For this review, take the finished solid that the model builds, in its own axes (mm). Face numbers are marked on the shaded views. A direction names the side the tool comes from. Round coordinates to 2 decimals unless told otherwise and drop trailing zeros. Order: outer loops, then holes, each group sorted by start corner. A loop starts at its lowest first (then second) coordinate and runs counter-clockwise, first axis right, second up.
from build123d import *

# Parameters (mm, degrees)
SKETCH1_W           = 26
SKETCH1_H           = 45
BOSS_EXTRUDE1_DEPTH = 11
SKETCH2_R           = 8.45
CUT_EXTRUDE1_DEPTH  = 28
CUT_EXTRUDE2_DEPTH  = 26.5
SKETCH5_W           = 6
SKETCH5_H           = 3
CUT_EXTRUDE3_DEPTH  = 53.509522946
BOSS_EXTRUDE4_START = 19
BOSS_EXTRUDE4_DEPTH = 19
SKETCH8_W           = 16
SKETCH8_H           = 16
CUT_EXTRUDE7_DEPTH  = 1.95
SKETCH9_W           = 6
SKETCH9_H           = 3
CUT_EXTRUDE8_DEPTH  = 53.502404707
SKETCH10_R          = 2
CUT_EXTRUDE9_DEPTH  = 4
SKETCH11_R          = 1.3
BOSS_EXTRUDE5_DEPTH = 26
SKETCH13_W          = 22
SKETCH13_H          = 12.79225404
CUT_EXTRUDE11_DEPTH = 54.122499941


with BuildPart() as part:
    # Sketch1 → Boss-Extrude1 (new body)
    with BuildSketch(Plane.XY):
        with Locations((13, -22.5)):
            Rectangle(SKETCH1_W, SKETCH1_H)
    extrude(amount=BOSS_EXTRUDE1_DEPTH)

    # Sketch2 → Cut-Extrude1 (cut)
    with BuildSketch(Plane.XZ.offset(45)):
        with Locations((13, -5.95)):
            Circle(SKETCH2_R)
    extrude(amount=-CUT_EXTRUDE1_DEPTH, mode=Mode.SUBTRACT)

    # Sketch4 → Cut-Extrude2 (cut)
    with BuildSketch(Plane(origin=(0, -43.5, 0), x_dir=(-1, 0, 0), z_dir=(0, -1, 0))):
        with BuildLine():
            Line((-1, -11), (-1, -1))
            Line((-1, -1), (-6.596875763, -1))
            ThreePointArc((-6.596875763, -1), (-13, -3.5), (-19.403124237, -1))
            Line((-19.403124237, -1), (-25, -1))
            Line((-25, -1), (-25, -11))
            Line((-25, -11), (-1, -11))
        make_face()
    extrude(amount=-CUT_EXTRUDE2_DEPTH, mode=Mode.SUBTRACT)

    # Sketch5 → Cut-Extrude3 (cut, through all)
    with BuildSketch(Plane.XY.offset(3.5)):
        with Locations((13, -26.5)):
            Rectangle(SKETCH5_W, SKETCH5_H)
    extrude(amount=-CUT_EXTRUDE3_DEPTH, mode=Mode.SUBTRACT)

    # Sketch6 → Boss-Extrude4 (add)
    with BuildSketch(Plane.XZ.offset(17).offset(BOSS_EXTRUDE4_START)):
        with BuildLine():
            Line((6.596875763, 1), (3.5, 1))
            Line((3.5, 1), (3.5, 5.5))
            Line((3.5, 5.5), (22.5, 5.5))
            Line((22.5, 5.5), (22.5, 1))
            Line((22.5, 1), (19.403124237, 1))
            ThreePointArc((19.403124237, 1), (13, 3.5), (6.596875763, 1))
        make_face()
    extrude(amount=-BOSS_EXTRUDE4_DEPTH)

    # Sketch8 → Cut-Extrude7 (cut)
    with BuildSketch(Plane.XY.offset(5.5)):
        with Locations((13, -26.5)):
            Rectangle(SKETCH8_W, SKETCH8_H)
    extrude(amount=-CUT_EXTRUDE7_DEPTH, mode=Mode.SUBTRACT)

    # Sketch9 → Cut-Extrude8 (cut, through all)
    with BuildSketch(Plane.XY.offset(3.55)):
        with Locations((13, -26.5)):
            Rectangle(SKETCH9_W, SKETCH9_H)
    extrude(amount=-CUT_EXTRUDE8_DEPTH, mode=Mode.SUBTRACT)

    # Sketch10 → Cut-Extrude9 (cut)
    with BuildSketch(Plane(origin=(26, 0, 0), x_dir=(0, 0, -1), z_dir=(1, 0, 0))):
        with Locations(Location((-5.5, -39, 0), (0, 0, 90))):
            Circle(SKETCH10_R)
    extrude(amount=-CUT_EXTRUDE9_DEPTH, mode=Mode.SUBTRACT)

    # Sketch11 → Boss-Extrude5 (add)
    with BuildSketch(Plane(origin=(26, 0, 0), x_dir=(0, 0, -1), z_dir=(1, 0, 0))):
        with BuildLine():
            Line((0, -10), (3, -10))
            ThreePointArc((3, -10), (6, -13), (3, -16))
            Line((3, -16), (0, -16))
            Line((0, -16), (0, -10))
        make_face()
        with Locations(Location((3, -13, 0), (0, 0, 90))):
            Circle(SKETCH11_R, mode=Mode.SUBTRACT)
    extrude(amount=-BOSS_EXTRUDE5_DEPTH)

    # Sketch13 → Cut-Extrude11 (cut, through all)
    with BuildSketch(Plane(origin=(0, 0, 0), x_dir=(-1, 0, 0), z_dir=(0, 0, -1))):
        with Locations((-13, -11.769971003)):
            Rectangle(SKETCH13_W, SKETCH13_H)
    extrude(amount=CUT_EXTRUDE11_DEPTH, mode=Mode.SUBTRACT)


solid = part.part
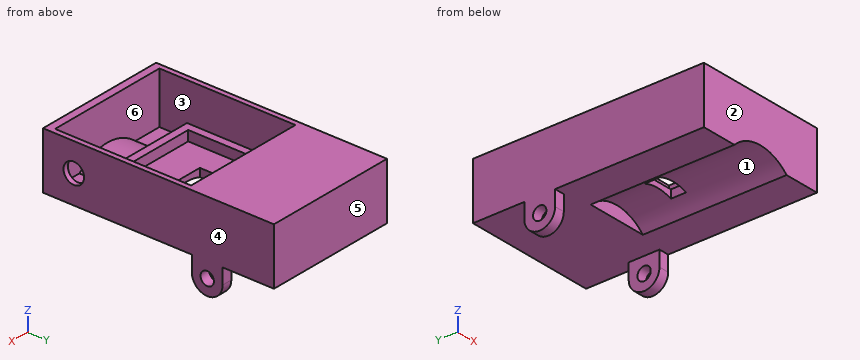
(1) Add section C-C on y = -39. Give the boundary of the cut face in (x, z).
(2) Clearance check with flat-ended pins moving along their axes: P1, Ø3, axis at x = 12, y = -38, coming from the -Z side; P2, Ø10, axis at y = -8.5, z = -2, coming from the +X side; P3, Ø8, axis at x = 22, y = -6.5, coming from the -Z side; P4, Ø0.6, axis at x = 25.5, z = -1, coming from the -Y side. State where each tip first meets the part, or that it passes through.
(3) Add section B-B on x = 13. Give the boundary of the cut face in (y, z).
(4) Add section A-A on y = -13. Give the boundary of the cut face in (x, z).
(5) Tool access review of the marked faces 1, 2 and 3: name each direction out of +Z, -Z, +X, -X, +Y, -Y from which nothing blocks a thin tool from reaching the whole face with its end or side.
(6) Wall thickness on L1, parallel to Y at x = 9.75, z = 5; L2, parallel to X at y = -35, z = 3.25; L3, parallel to X at y = -20.5, z = 3.75: over which ranges is each line inside the solid? List them lowest first.
(7) Add section D-D on z = -3.75. Give the boundary of the cut face in (x, y), plus the area to 3 significant figures.
(8) Draft analysis for pull direction Y (two halves, no side actions). For the marked faces 4, 5 and 6, state which applies: pulls with the +Y half, pulls with the -Y half, needs draft (parallel to the pull), parting line crosses it, or undercut.
Here are the results:
1. outline: (0, 0) - (7, 0) arc R8.45 cw to (19, 0) - (26, 0) - (26, 3.5) - (25, 3.5) - (25, 1) - (19.4, 1) arc R9.45 ccw to (6.6, 1) - (1, 1) - (1, 11) - (0, 11) - close; (25, 7.5) - (26, 7.5) - (26, 11) - (25, 11) - close
2. P1: stops at z = 2.12
2. P2: stops at x = 26
2. P3: stops at z = 0
2. P4: stops at y = -16
3. outline: (-45, 2.5) - (-28, 2.5) - (-28, 3.55) - (-34.5, 3.55) - (-34.5, 5.5) - (-36, 5.5) - (-36, 3.5) - (-43.5, 3.5) - (-43.5, 11) - (-45, 11) - close; (-25, 2.5) - (-17, 2.5) - (-17, 0) - (0, 0) - (0, 11) - (-17, 11) - (-17, 5.5) - (-18.5, 5.5) - (-18.5, 3.55) - (-25, 3.55) - close
4. outline: (0, -6) - (2, -6) - (2, -4.3) - (0, -4.3) - close; (0, -1.7) - (2, -1.7) - (2, 0) - (24, 0) - (24, -1.7) - (26, -1.7) - (26, 11) - (0, 11) - close; (24, -6) - (26, -6) - (26, -4.3) - (24, -4.3) - close
5. face 1: -Z, -Y
5. face 2: +Z, -Z, +X, -X, -Y
5. face 3: +Z
6. L1: y = -45 to -43.5, -36 to -34.5, -18.5 to 0
6. L2: x = 0 to 1, 3.5 to 22.5, 25 to 26
6. L3: x = 0 to 1, 3.5 to 5, 21 to 22.5, 25 to 26
7. outline: (0, -15.9) - (2, -15.9) - (2, -14.06) - (0, -14.06) - close; (0, -11.94) - (2, -11.94) - (2, -10.1) - (0, -10.1) - close; (24, -15.9) - (26, -15.9) - (26, -14.06) - (24, -14.06) - close; (24, -11.94) - (26, -11.94) - (26, -10.1) - (24, -10.1) - close
7. area: 14.7 mm2
8. face 4: needs draft
8. face 5: pulls with the +Y half
8. face 6: undercut
